Model file for the job. Use its own axes, mm. A direction names the side the tool comes from. Round coordinates to 2 decimals unless told otherwise and drop trailing zeros. Order: outer loops, then holes, each group sorted by start corner. A loop starts at its lowest first (then second) coordinate and runs counter-clockwise, first axis right, second up. Notation, with made-up numbers: (-0.75, 89.5) -> (25.25, 89.5) arc R32 ccw to (25.25, 122.5) -> close; hole circle Ø2 at (79, 39). An arc over 180 degrees is marked (long way). Use CSV: the item, a comma, the result in double quotes.
```python
from build123d import *

# Parameters (mm, degrees)
F0_R     = 30
F0_W     = 26
F0_H     = 26
F1_DEPTH = 3
F0_W_2   = 20
F0_H_2   = 20
F2_DEPTH = 25
F3_R     = 1
F5_D     = 3


with BuildPart() as f1:
    # F0 (on Top) → F1 (new body)
    with BuildSketch(Plane.XY):
        with Locations((10, 10)):
            Circle(F0_R)
        with Locations((10, 10)):
            Rectangle(F0_W, F0_H, mode=Mode.SUBTRACT)
    extrude(amount=-F1_DEPTH)

    # F0 (on Top) → F2 (join)
    with BuildSketch(Plane.XY):
        with Locations((10, 10)):
            Rectangle(F0_W, F0_H)
        with Locations((10, 10)):
            Rectangle(F0_W_2, F0_H_2, mode=Mode.SUBTRACT)
    extrude(amount=-F2_DEPTH)

    # F3
    f3_edges = [f1.edges().sort_by_distance(p)[0] for p in [
        (-20, 10, -3),
        (10, -3, -3),
        (-3, 10, -3),
        (10, 23, -3),
        (23, 10, -3),
        (-3, 23, -14),
        (10, 23, -25),
        (23, 23, -14),
        (23, 10, -25),
        (23, -3, -14),
        (10, -3, -25),
        (-3, -3, -14),
        (-3, 10, -25),
    ]]
    fillet(f3_edges, radius=F3_R)

    # F5 (through all)
    with Locations(Plane.XY):
        with Locations((10, 30), (30, 10), (10, -10), (-10, 10)):
            Hole(F5_D / 2)


solid = f1.part
```
Q1. Pin check, flat tips, straight feed: pin 1 (4 mm diameter, centred on x = 23, z = -7, fed in from +Y); pin 2 (1.5 mm diameter, centred on y = 13, z = -14.5, fed in from -X); pin 3 (6 mm diameter, centred on y = 10.5, z = -10.5, fed in from +X). Stop position of each tip, or through.
From the geometry:
pin 1,"stops at y = 23"
pin 2,"stops at x = -3"
pin 3,"stops at x = 23"
Q2. Probe line 1 along Y through (x, z) = (10, -1.4); line 2 along Y through (x, z) = (8, -23.5). List the from-to ranges inside material, lowest first.
From the geometry:
line 1,"y = -20 to -11.5, -8.5 to 0, 20 to 28.5, 31.5 to 40"
line 2,"y = -3 to 0, 20 to 23"
Q3. Which spindle directions (+Z, -Z, +X, -X, +Y, -Y) get a long thin tool onto all of the face, cutting with end or side? Do faces 4 (the flat face through (10, 20, -12)), 5 (the flat face through (-3, 10, -14)), 6 (the flat face through (23, 10, -14)). Say none if no direction does.
From the geometry:
face 4,"+Z, -Z"
face 5,"-Z, -X, +Y, -Y"
face 6,"-Z, +X, +Y, -Y"
Q4. Cut at A-A (y = 10). Give the cut face in (x, z), plus the area to 3 significant figures.
From the geometry:
outline,"(-20, -2) arc R1 ccw to (-19, -3) -> (-11.5, -3) -> (-11.5, 0) -> (-20, 0) -> close; (-8.5, -3) -> (-4, -3) arc R1 cw to (-3, -4) -> (-3, -24) arc R1 ccw to (-2, -25) -> (0, -25) -> (0, 0) -> (-8.5, 0) -> close; (20, -25) -> (22, -25) arc R1 ccw to (23, -24) -> (23, -4) arc R1 cw to (24, -3) -> (28.5, -3) -> (28.5, 0) -> (20, 0) -> close; (31.5, -3) -> (39, -3) arc R1 ccw to (40, -2) -> (40, 0) -> (31.5, 0) -> close"
area,"234 mm²"
Q5. Cut at B-B (z = -17). Give the cut face in (x, y), plus the area to 3 significant figures.
From the geometry:
outline,"(-3, -2) arc R1 ccw to (-2, -3) -> (22, -3) arc R1 ccw to (23, -2) -> (23, 22) arc R1 ccw to (22, 23) -> (-2, 23) arc R1 ccw to (-3, 22) -> close; hole (0, 0) -> (20, 0) -> (20, 20) -> (0, 20) -> close"
area,"275 mm²"
Q6. Mould opens along Y. For faces 1 (the cylindrical face through (11.2, -10.9, -1.5)), 2 (the flat face through (10, 23, -14)), 3 (the cylindrical face through (-12.111, 30.275, -0.986)) say: +Y half, -Y half, draft (parallel to the pull), parting line (faces both ways), or undercut.
From the geometry:
face 1,"undercut"
face 2,"+Y half"
face 3,"parting line"
